Autodesk Inventor part; units mm, degrees
ref_plane "YZ Plane" through (0, 0, 0) normal (1, 0, 0) x (0, 1, 0)
ref_plane "XZ Plane" through (0, 0, 0) normal (0, 1, 0) x (-1, 0, 0)
ref_plane "XY Plane" through (0, 0, 0) normal (0, 0, 1) x (1, 0, 0)
sketch "Sketch_1" plane through (0, 0, 0) normal (0, 0, 1) x (1, 0, 0)
  arc A0 (-19.05, 3.175) -> (-15.875, 0) centre (-15.875, 3.175) ccw
  line L0 (-15.875, 0) -> (15.875, 0)
  arc A1 (15.875, 0) -> (19.05, 3.175) centre (15.875, 3.175) ccw
  line L1 (19.05, 3.175) -> (19.05, 15.875)
  arc A2 (19.05, 15.875) -> (15.875, 19.05) centre (15.875, 15.875) ccw
  line L2 (15.875, 19.05) -> (5.6388, 19.05)
  arc A3 (5.6388, 19.05) -> (4.064, 17.4752) centre (5.6388, 17.4752) ccw
  line L3 (4.064, 17.4752) -> (4.064, 16.5608)
  arc A4 (4.064, 16.5608) -> (5.6388, 14.986) centre (5.6388, 16.5608) ccw
  line L4 (5.6388, 14.986) -> (9.398, 14.986)
  arc A5 (10.287, 14.097) -> (9.398, 14.986) centre (9.398, 14.097) ccw
  line L5 (10.287, 14.097) -> (10.287, 13.7794)
  arc A6 (10.0266, 13.1508) -> (10.287, 13.7794) centre (9.398, 13.7794) ccw
  line L6 (10.0266, 13.1508) -> (5.125, 8.2492)
  arc A7 (1.7664, 6.858) -> (5.125, 8.2492) centre (1.7664, 11.6078) ccw
  line L7 (1.7664, 6.858) -> (-1.7664, 6.858)
  arc A8 (-5.125, 8.2492) -> (-1.7664, 6.858) centre (-1.7664, 11.6078) ccw
  line L8 (-5.125, 8.2492) -> (-10.0266, 13.1508)
  arc A9 (-10.287, 13.7794) -> (-10.0266, 13.1508) centre (-9.398, 13.7794) ccw
  line L9 (-10.287, 13.7794) -> (-10.287, 14.097)
  arc A10 (-9.398, 14.986) -> (-10.287, 14.097) centre (-9.398, 14.097) ccw
  line L10 (-9.398, 14.986) -> (-5.6388, 14.986)
  arc A11 (-5.6388, 14.986) -> (-4.064, 16.5608) centre (-5.6388, 16.5608) ccw
  line L11 (-4.064, 16.5608) -> (-4.064, 17.4752)
  arc A12 (-4.064, 17.4752) -> (-5.6388, 19.05) centre (-5.6388, 17.4752) ccw
  line L12 (-5.6388, 19.05) -> (-15.875, 19.05)
  arc A13 (-15.875, 19.05) -> (-19.05, 15.875) centre (-15.875, 15.875) ccw
  line L13 (-19.05, 15.875) -> (-19.05, 3.175)
  circle A14 centre (14.8488, 14.8014) radius 2.5527
  circle A15 centre (12.7, 6.35) radius 3.3274
  circle A16 centre (-12.7, 6.35) radius 3.3274
  circle A17 centre (-14.8488, 14.8014) radius 2.5527
extrude "Extrusion1" add sketch "Sketch_1" against normal blind 584.2
properties part number "Cross Brace"
Here's how the part is built. I have some questions about the finished solid (model axes, mm). Round coordinates to 2 decimals unless told otherwise and drop trailing zeros.
1. If we section it at A-A on z = -96: Count the separate pieces of the cut face and the enclosed holes in it, plus the area to 3 significant figures.
Answer list:
separate pieces: 1
enclosed holes: 4
area: 449 mm2
2. If I drill on line 1 along X through (y, z) = (6.5, -502.5); line 2 along Y through (x, z) = (-13.5, -42.5); line 3 along Y through (x, z) = (13, -537.5), over which ranges is the centre line in solid material (lowest first)?
Answer list:
line 1: x = -19.05 to -16.02, -9.38 to 9.38, 16.02 to 19.05
line 2: y = 0 to 3.12, 9.58 to 12.63, 16.97 to 19.05
line 3: y = 0 to 3.04, 9.66 to 13.04, 16.56 to 19.05
3. For P1, Ø1, axis at x = -15, z = -242.5, coming from the -Y side; P2, Ø0.7, axis at y = 17, z = -289.5, coming from the +X side; P3, Ø3, axis at x = 1, z = -205, coming from the +Y side (3 decimals); P4, Ø1, axis at x = 1.5, y = 8.5, coming from the -Z side, each with a flat end and sliding along its axis, tell me the tip position at first contact or that it passes through.
Answer list:
P1: stops at y = 0
P2: stops at x = 18.95
P3: stops at y = 6.915
P4: passes through
